```python
from build123d import *

# Parameters (mm, degrees)
SKETCH1_R      = 12.7
EXTRUDE1_DEPTH = 25.4


with BuildPart() as part:
    # Sketch1 → Extrude1 (new body)
    with BuildSketch(Plane(origin=(0, 0, 0), x_dir=(1, 0, 0), z_dir=(0, 1, 0))):
        with BuildLine():
            ThreePointArc((-15.009090909, 61.700706561), (-60.542428713, -19.15370266), (23.210344828, -59.106090151))
            ThreePointArc((23.210344828, -59.106090151), (74.601523764, -43.982890719), (127.846666667, -38.090591431))
            ThreePointArc((127.846666667, -38.090591431), (163.49081416, -10.955842364), (148.687692308, 31.3249741))
            ThreePointArc((148.687692308, 31.3249741), (70.093122075, 64.047893785), (-15.009090909, 61.700706561))
        make_face()
        with Locations(Location((50.8, 6.35, 0), (0, 0, 270))):
            Circle(SKETCH1_R, mode=Mode.SUBTRACT)
        with BuildLine():
            Line((-43.815, 13.97), (-32.385, 13.97))
            ThreePointArc((-32.385, 13.97), (-28.575, 6.35), (-32.385, -1.27))
            Line((-32.385, -1.27), (-43.815, -1.27))
            ThreePointArc((-43.815, -1.27), (-47.625, 6.35), (-43.815, 13.97))
        make_face(mode=Mode.SUBTRACT)
    extrude(amount=EXTRUDE1_DEPTH)


solid = part.part
```
The model under review builds one solid part; all positions refer to its coordinate system, in mm. A direction names the side the tool comes from. Round coordinates to 2 decimals unless told otherwise and drop trailing zeros. Loops run counter-clockwise (first coordinate to the right, second up) from the corner with the lowest first, then second, coordinate; pieces in that order, holes last. Notation, with made-up numbers: (7, 18) -> (17, 18) arc R21 cw to (17, 49) -> close; hole circle Ø5 at (2.25, 27.25). An arc over 180 degrees is marked (long way). Answer as a JSON object with one key per item and string values. Group by question number.
1) We need section C-C on z = -6.35. Write out the cut boundary in (x, y) (3 decimals), then the cut area to 3 significant figures.
2) We need section B-B on x = 41. Write out the cut boundary in (y, z), then the cut area to 3 significant figures.
3) We need section A-A on y = 13.25. Write out the cut boundary in (x, z) (3 decimals).
4) For faces 1 (the face through (-47.624, 12.522, -6.226)), 2 (the face through (24, 0, -3)), list the 3-axis set-ups (+Z, -Z, +X, -X, +Y, -Y) from which the entire face can be reached by the end or side of a thin tool; tool diameter is ignored.
5) Mouldability with a two-part tool opening along Z and no side actions: class faces 3 (the face through (24, 25.4, -3)), 4 (the face through (-38, 13, 1.27)), 5 (the face through (-60.966, 12.522, 17.76)) as released by +Z, released by -Z, zero draft, split by the parting line, or undercut.
6) For line 1 (Z direction, x = -30, y = 21.5); line 2 (X direction, y = 6, z = -16); line 3 (X direction, y = 13.25, z = -42.5), list the stretches that pass through material, from the lowest coordinate up. Write a range as [from, to].
7) We need section D-D on z = -45. Write out the cut boundary in (x, y).
8) For pin 1 Ø9 at (x, y) = (-38.5, 11.5) entering from -Z; pin 2 Ø8 at (y, z) = (14, 26.5) entering from +X; pin 3 Ø12 at (y, z) = (9.5, -10.5) entering from +X; pin 4 Ø15 at (x, z) = (50.8, -6.35) entering from -Y, all flat-tipped, find the tip position at first contact; note any pin that passes through.
Result set:
{
 "1": {"outline": "(-63.182, 0) -> (-47.625, 0) -> (-47.625, 25.4) -> (-63.182, 25.4) -> close; (-28.575, 0) -> (38.1, 0) -> (38.1, 25.4) -> (-28.575, 25.4) -> close; (63.5, 0) -> (164.567, 0) -> (164.567, 25.4) -> (63.5, 25.4) -> close", "area": "4,660 mm²"},
 "2": {"outline": "(0, -67.3) -> (25.4, -67.3) -> (25.4, -14.43) -> (0, -14.43) -> close; (0, 1.73) -> (25.4, 1.73) -> (25.4, 52.75) -> (0, 52.75) -> close", "area": "2,640 mm²"},
 "3": {"outline": "(-15.009, -61.701) arc R203.2 ccw to (148.688, -31.325) arc R38.1 ccw to (127.847, 38.091) arc R304.8 cw to (23.21, 59.106) arc R63.5 ccw (long way) to start; hole (-43.815, -13.97) -> (-32.385, -13.97) arc R9.525 ccw to (-32.385, 1.27) -> (-43.815, 1.27) arc R9.525 ccw to start; hole circle Ø25.4 at (50.8, -6.35)"},
 "4": {"face 1": "+Y, -Y", "face 2": "+Z, -Z, +X, -X, -Y"},
 "5": {"face 3": "zero draft", "face 4": "undercut", "face 5": "split by the parting line"},
 "6": {"line 1": "[-55.97, -11.36], [-1.34, 55.97]", "line 2": "[-61.45, 42.54], [59.06, 161.58]", "line 3": "[-47.18, 130.59]"},
 "7": {"outline": "(-44.8, 0) -> (125.88, 0) -> (125.88, 25.4) -> (-44.8, 25.4) -> close"},
 "8": {"pin 1": "z = -53.63", "pin 2": "x = 157.75", "pin 3": "x = 164.83", "pin 4": "through"}
}
